Read the model definition and answer for the solid it produces. Units are mm, in the model's axes. Face numbers are marked on the shaded views. A direction names the side the tool comes from. Coordinates: 2 decimals unless noted, no trailing zeros. Order: outer loops, then holes, each group sorted by start corner. A loop starts at its lowest first (then second) coordinate and runs counter-clockwise, first axis right, second up. Notation, with made-up numbers: (61, -22.5) -> (77, -22.5) arc R22 cw to (77, -1.5) -> close; hole circle Ø5 at (68.5, 0.5). An arc over 180 degrees is marked (long way). Answer in a Markdown table with one row per item.
from build123d import *

# Parameters (mm, degrees)
EXTRUDE_319_DEPTH   = 30
EXTRUDE_1_DEPTH     = 30
SKETCH_3_R          = 5
CUT_EXTRUDE_1_DEPTH = 50.558046773
CUT_EXTRUDE_2_DEPTH = 5


with BuildPart() as part:
    # Эскиз1 → Extrude 319 (new body)
    with BuildSketch(Plane(origin=(0, 0, 0), x_dir=(1, 0, 0), z_dir=(0, 1, 0))):
        Polygon((20, 0), (-20, 0), (-20, 34), (-15, 34), (-2.5, 21.5), (-2.5, 16.5), (2.5, 16.5), (2.5, 21.5), (15, 34), (20, 34), align=None)
    extrude(amount=EXTRUDE_319_DEPTH)

    # Эскиз2 → Бобышка-Вытянуть1 (add)
    with BuildSketch(Plane(origin=(0, 30, 0), x_dir=(-1, 0, 0), z_dir=(0, 1, 0))):
        with BuildLine():
            Line((10, 0), (-10, 0))
            ThreePointArc((-10, 0), (0, 10), (10, 0))
        make_face()
    extrude(amount=-EXTRUDE_1_DEPTH)

    # Эскиз3 → Вырез-Вытянуть1 (cut, through all)
    with BuildSketch(Plane(origin=(0, 30, 0), x_dir=(-1, 0, 0), z_dir=(0, 1, 0))):
        with Locations(Location((0, 0, 0), (0, 0, 90))):
            Circle(SKETCH_3_R)
    extrude(amount=-CUT_EXTRUDE_1_DEPTH, mode=Mode.SUBTRACT)

    # Эскиз4 → Вырез-Вытянуть2 (cut)
    with BuildSketch(Plane(origin=(0, 30, 0), x_dir=(-1, 0, 0), z_dir=(0, 1, 0))):
        with BuildLine():
            Line((-10, 0), (-20, 0))
            Line((-20, 0), (-20, -14))
            Line((-20, -14), (20, -14))
            Line((20, -14), (20, 0))
            Line((20, 0), (10, 0))
            ThreePointArc((10, 0), (0, 10), (-10, 0))
        make_face()
    extrude(amount=-CUT_EXTRUDE_2_DEPTH, mode=Mode.SUBTRACT)


solid = part.part
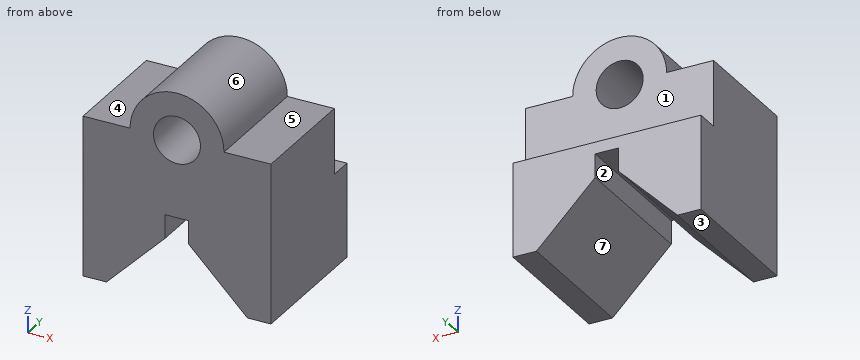
Q1. The part is cut by section A-A (z = -29). Write down the section's boundary in (x, y).
Outcome:
| item | result |
|---|---|
| outline | (-20, 0) -> (-10, 0) -> (-10, 30) -> (-20, 30) -> close; (10, 0) -> (20, 0) -> (20, 30) -> (10, 30) -> close |
Q2. The part is cut by section C-C (x = 0). Write down the section's boundary in (y, z).
Outcome:
| item | result |
|---|---|
| outline | (0, -16.5) -> (30, -16.5) -> (30, -14) -> (25, -14) -> (25, -5) -> (0, -5) -> close; (0, 5) -> (25, 5) -> (25, 10) -> (0, 10) -> close |
Q3. For the marked faces 1, 2, 3 and 4, determine the directions among +Z, -Z, +X, -X, +Y, -Y from which every point of the face is accessible in a straight line to the end or side of a thin tool.
Outcome:
| item | result |
|---|---|
| face 1 | +Z, +X, -X, +Y |
| face 2 | -Z, +Y, -Y |
| face 3 | -Z, +X, -X, +Y, -Y |
| face 4 | +Z, -X, +Y, -Y |
Q4. The part is cut by section B-B (y = 13.75). Write down the section's boundary in (x, z).
Outcome:
| item | result |
|---|---|
| outline | (-20, -34) -> (-15, -34) -> (-2.5, -21.5) -> (-2.5, -16.5) -> (2.5, -16.5) -> (2.5, -21.5) -> (15, -34) -> (20, -34) -> (20, 0) -> (10, 0) arc R10 ccw to (-10, 0) -> (-20, 0) -> close; hole circle Ø10 at (0, 0) |
Q5. For a pull along X with two mould halves and no side action, classify the marked faces 5, 6 and 7 as pulls with the +X half, pulls with the -X half, needs draft (parallel to the pull), parting line crosses it, or undercut.
Outcome:
| item | result |
|---|---|
| face 5 | needs draft |
| face 6 | parting line crosses it |
| face 7 | undercut |
Q6. Given pin 1 (1.5 mm diameter, centred on x = -9, y = 27, fed in from +Z); pin 2 (2 mm diameter, centred on x = -3.5, y = 20, fed in from -Z); pin 3 (1 mm diameter, centred on x = -5, z = -3.5, fed in from +Y), each flat-ended and moving along its own axis, determine where each tip first touches the part or whether it passes through.
Outcome:
| item | result |
|---|---|
| pin 1 | z = -14 |
| pin 2 | z = -23.5 |
| pin 3 | y = 25 |
Q7. Consider line 1 (X direction, y = 24.5, z = -18.5); line 2 (Y direction, x = 11, z = -6); line 3 (Z direction, x = 17, y = 27.5). Determine where each line is inside the solid, lowest interval first.
Outcome:
| item | result |
|---|---|
| line 1 | -20 to -2.5, 2.5 to 20 |
| line 2 | 0 to 25 |
| line 3 | -34 to -14 |
Q8. The part is cut by section D-D (z = -19). Write down the section's boundary in (x, y).
Outcome:
| item | result |
|---|---|
| outline | (-20, 0) -> (-2.5, 0) -> (-2.5, 30) -> (-20, 30) -> close; (2.5, 0) -> (20, 0) -> (20, 30) -> (2.5, 30) -> close |
